Verification items for the finished model (mm, model axes). A direction names the side the tool comes from. Give positions to 0.01 mm unless a question says otherwise; leave off trailing zeros. Order: outer loops, then holes, each group sorted by start corner. A loop starts at its lowest first (then second) coordinate and runs counter-clockwise, first axis right, second up.
(1) Sectioned sample at B-B on y = -7. Record the cut outline in (x, z), plus the area to 3 significant figures.
(2) Scan lines: L1, parallel to Z at x = -1.05, y = 5.5; L2, parallel to Z at x = -1.1, y = 6.75; L3, parallel to Z at x = 0, y = -6.5. Record each from-to range of solid material in increasing order.
(3) Mould release check, pull along Z, two halves, no side actions. Record for faces 4 (the face through (0, 8, 77)), 5 (the face through (0, 6, 55)), 6 (the face through (0, -7, 100)), 7 (the face through (0, 5, 50)): pulls with the +Z half, pulls with the -Z half, needs draft (parallel to the pull), parting line crosses it, or undercut.
(4) Sectioned sample at A-A on x = 0.5. Record the cut outline in (y, z).
(5) Access from +Z, -Z, +X, -X, +Y, -Y to the whole of each face (thin tool, end or side, straight path). Record for faces 1 (the face through (0, 6, 45)), 2 (the face through (0, -6, -1)), 3 (the face through (0, -6, 101)).
(6) Gauge pin test, flat ends, axial feed: pin 1 (1.2 mm diameter, centred on x = 0.5, z = -1, fed in from +Y); pin 2 (0.8 mm diameter, centred on x = 0, z = 51, fed in from +Y); pin 3 (0.6 mm diameter, centred on x = 0.5, y = -7, fed in from +Z). Record the tip position at first contact, or that the pin passes through.
```python
from build123d import *

# Parameters (mm, degrees)
SKETCH1_W           = 2.5
SKETCH1_H           = 16
BOSS_EXTRUDE1_DEPTH = 100
SKETCH1_3_W         = 2.5
SKETCH1_3_H         = 12
BOSS_EXTRUDE2_DEPTH = 3
SKETCH2_W           = 10
SKETCH2_H           = 3
CUT_EXTRUDE1_DEPTH  = 10


with BuildPart() as part:
    # Sketch1 → Boss-Extrude1 (new body)
    with BuildSketch(Plane.XY):
        Rectangle(SKETCH1_W, SKETCH1_H)
    extrude(amount=BOSS_EXTRUDE1_DEPTH)

    # Sketch1<3> → Boss-Extrude2 (add)
    with BuildSketch(Plane.XY):
        Rectangle(SKETCH1_3_W, SKETCH1_3_H)
    boss_extrude2 = extrude(amount=-BOSS_EXTRUDE2_DEPTH)

    # Mirror1: Boss-Extrude2 across plane
    add(boss_extrude2.mirror(Plane(origin=(0, 0, 50), x_dir=(1, 0, 0), z_dir=(0, 0, -1))))

    # Sketch2 → Cut-Extrude1 (cut)
    with BuildSketch(Plane(origin=(1.25, 0, 0), x_dir=(0, 0, -1), z_dir=(1, 0, 0))):
        with Locations((-50, 6.5)):
            Rectangle(SKETCH2_W, SKETCH2_H)
    extrude(amount=-CUT_EXTRUDE1_DEPTH, mode=Mode.SUBTRACT)


solid = part.part
```
Ans:
1. outline: (-1.25, 0) - (1.25, 0) - (1.25, 100) - (-1.25, 100) - close
1. area: 250 mm2
2. L1: z = -3 to 45, 55 to 103
2. L2: z = 0 to 45, 55 to 100
2. L3: z = 0 to 100
3. face 4: needs draft
3. face 5: undercut
3. face 6: pulls with the +Z half
3. face 7: undercut
4. outline: (-8, 0) - (-6, 0) - (-6, -3) - (6, -3) - (6, 0) - (8, 0) - (8, 45) - (5, 45) - (5, 55) - (8, 55) - (8, 100) - (6, 100) - (6, 103) - (-6, 103) - (-6, 100) - (-8, 100) - close
5. face 1: +X, -X, +Y
5. face 2: -Z, +X, -X, -Y
5. face 3: +Z, +X, -X, -Y
6. pin 1: stops at y = 6
6. pin 2: stops at y = 5
6. pin 3: stops at z = 100
